Input: part model. Units: mm. Frame: model coordinates. A direction names the side the tool comes from. Give positions to 0.01 mm unless a question says otherwise; leave off trailing zeros. Loops run counter-clockwise (first coordinate to the right, second up) from the corner with the lowest first, then second, coordinate; pieces in that order, holes last. Notation, with made-up numbers: M 28,31 L 76,31 A12 ccw 76,53 Z; hole C -6,-24 d3. An arc over 180 degrees is marked long. Use CSV: the item, a comma, the result in double quotes. Start each with the question number.
Q1. Material intervals for line 1 along Z through (x, y) = (31, 13.5); line 2 along Y through (x, z) = (-48, 21.5); line 3 along Y through (x, z) = (-24, 26), sorted ascending.
Q2. Section B-B, the plane y = 25. Output: boundary loops of the cut face in (x, z).
Q3. Section A-A, the plane x = 0. Output: boundary loops of the cut face in (y, z), plus the area to 3 significant figures.
Q4. Section C-C, the plane x = 24. Output: boundary loops of the cut face in (y, z), plus the area to 3 significant figures.
Q5. Section D-D, the plane y = 3.5. Output: boundary loops of the cut face in (x, z) (3 decimals).
Q6. Pull-direction query (Z, two-part tool) for faces 1 (the flat face through (-1, 22, 16.95)), 2 (the cylindrical face through (-13.59, 1.01, 7.15)), 3 (the cylindrical face through (-46.06, 13.2, 20.52)), 4 (the flat face through (-2, 16, -24)); classes: released by +Z, released by -Z, zero draft, split by the parting line, or undercut.
Q7. Pin query (flat end, axial travel): pin 1 (3.5 mm diameter, centred on x = -14.94, z = -8.62, fed in from -Y); pin 2 (9 mm diameter, centred on x = -14.94, z = -8.62, fed in from +Y); pin 3 (6 mm diameter, centred on x = -24, y = 14, fed in from +Z). Return the tip coordinate at first contact, or that it passes through.
Q8. Reachability of faces 5 (the flat face through (-1, 36, 22)), 6 (the flat face through (-1, 7, -8)), 7 (the flat face through (27, 15.8, -25.5)), 8 (the cylindrical face through (-21.997, 14.631, 20.524)), 9 (the flat face through (-46, 12, 24)) from +Z, -Z, +X, -X, +Y, -Y: full face, straight path, thin tool, end or side. Return the list, or none.
from build123d import *

# Parameters (mm, degrees)
SKETCH1_W           = 108
SKETCH1_H           = 54
BOSS_EXTRUDE1_DEPTH = 6
SKETCH2_R           = 2
CUT_EXTRUDE1_DEPTH  = 12
SKETCH3_R           = 3.5
CUT_EXTRUDE3_DEPTH  = 4
SKETCH4_W           = 108
SKETCH4_H           = 54
BOSS_EXTRUDE2_DEPTH = 30
SKETCH5_W           = 108
SKETCH5_H           = 33.9
CUT_EXTRUDE4_DEPTH  = 29
SKETCH6_R           = 2.1
CUT_EXTRUDE5_DEPTH  = 67
SKETCH7_R           = 3.6
CUT_EXTRUDE6_DEPTH  = 3
CUT_EXTRUDE7_DEPTH  = 3
CUT_EXTRUDE8_START  = -3
SKETCH10_R          = 3.5
CUT_EXTRUDE8_DEPTH  = 3
SKETCH11_R          = 4
CUT_EXTRUDE9_DEPTH  = 10


with BuildPart() as part:
    # Sketch1 → Boss-Extrude1 (new body)
    with BuildSketch(Plane(origin=(0, 0, 0), x_dir=(1, 0, 0), z_dir=(0, 1, 0))):
        Rectangle(SKETCH1_W, SKETCH1_H)
    extrude(amount=BOSS_EXTRUDE1_DEPTH)

    # Sketch2 → Cut-Extrude1 (cut)
    with BuildSketch(Plane(origin=(0, 6, 0), x_dir=(1, 0, 0), z_dir=(0, 1, 0))):
        with Locations(Location((-14.938938215, 8.625, 0), (0, 0, 270))):
            Circle(SKETCH2_R)
        with Locations(Location((-14.938938215, -8.625, 0), (0, 0, 270))):
            Circle(SKETCH2_R)
        with Locations(Location((15.385610645, 7.800351601, 0), (0, 0, 270))):
            Circle(SKETCH2_R)
        with Locations(Location((15.385610645, -8.625, 0), (0, 0, 270))):
            Circle(SKETCH2_R)
    extrude(amount=-CUT_EXTRUDE1_DEPTH, mode=Mode.SUBTRACT)

    # Sketch3 → Cut-Extrude3 (cut)
    with BuildSketch(Plane(origin=(0, 6, 0), x_dir=(1, 0, 0), z_dir=(0, 1, 0))):
        with Locations(Location((-14.938938215, 8.625, 0), (0, 0, 270))):
            Circle(SKETCH3_R)
        with Locations(Location((-14.938938215, -8.625, 0), (0, 0, 270))):
            Circle(SKETCH3_R)
        with Locations(Location((15.385610645, 7.800351601, 0), (0, 0, 270))):
            Circle(SKETCH3_R)
        with Locations(Location((15.385610645, -8.625, 0), (0, 0, 270))):
            Circle(SKETCH3_R)
    extrude(amount=-CUT_EXTRUDE3_DEPTH, mode=Mode.SUBTRACT)

    # Sketch4 → Boss-Extrude2 (add)
    with BuildSketch(Plane(origin=(0, 6, 0), x_dir=(1, 0, 0), z_dir=(0, 1, 0))):
        Rectangle(SKETCH4_W, SKETCH4_H)
    extrude(amount=BOSS_EXTRUDE2_DEPTH)

    # Sketch5 → Cut-Extrude4 (cut)
    with BuildSketch(Plane(origin=(0, 36, 0), x_dir=(1, 0, 0), z_dir=(0, 1, 0))):
        Rectangle(SKETCH5_W, SKETCH5_H)
    extrude(amount=-CUT_EXTRUDE4_DEPTH, mode=Mode.SUBTRACT)

    # Sketch6 → Cut-Extrude5 (cut)
    with BuildSketch(Plane.XY.offset(27)):
        with Locations((0, 14)):
            Circle(SKETCH6_R)
        with Locations((-24, 14)):
            Circle(SKETCH6_R)
        with Locations((-48, 14)):
            Circle(SKETCH6_R)
        with Locations((24, 14)):
            Circle(SKETCH6_R)
        with Locations((48, 14)):
            Circle(SKETCH6_R)
        with Locations((48, 32)):
            Circle(SKETCH6_R)
        with Locations((-48, 32)):
            Circle(SKETCH6_R)
    extrude(amount=-CUT_EXTRUDE5_DEPTH, mode=Mode.SUBTRACT)

    # Sketch7 → Cut-Extrude6 (cut)
    with BuildSketch(Plane.XY.offset(27)):
        with Locations((-48, 32)):
            Circle(SKETCH7_R)
        with Locations((-48, 14)):
            Circle(SKETCH7_R)
        with Locations((-24, 14)):
            Circle(SKETCH7_R)
        with Locations((0, 14)):
            Circle(SKETCH7_R)
        with Locations((24, 14)):
            Circle(SKETCH7_R)
        with Locations((48, 14)):
            Circle(SKETCH7_R)
        with Locations((48, 32)):
            Circle(SKETCH7_R)
    extrude(amount=-CUT_EXTRUDE6_DEPTH, mode=Mode.SUBTRACT)

    # Sketch8 → Cut-Extrude7 (cut)
    with BuildSketch(Plane(origin=(0, 0, -27), x_dir=(-1, 0, 0), z_dir=(0, 0, -1))):
        Polygon((-50.020725942, 28.5), (-45.979274058, 28.5), (-43.958548116, 32), (-45.979274058, 35.5), (-50.020725942, 35.5), (-52.041451884, 32), align=None)
        Polygon((-50.020725942, 10.5), (-45.979274058, 10.5), (-43.958548116, 14), (-45.979274058, 17.5), (-50.020725942, 17.5), (-52.041451884, 14), align=None)
        Polygon((-26.020725942, 10.5), (-21.979274058, 10.5), (-19.958548116, 14), (-21.979274058, 17.5), (-26.020725942, 17.5), (-28.041451884, 14), align=None)
        Polygon((-2.020725942, 10.5), (2.020725942, 10.5), (4.041451884, 14), (2.020725942, 17.5), (-2.020725942, 17.5), (-4.041451884, 14), align=None)
        Polygon((21.979274058, 10.5), (26.020725942, 10.5), (28.041451884, 14), (26.020725942, 17.5), (21.979274058, 17.5), (19.958548116, 14), align=None)
        Polygon((45.979274058, 10.5), (50.020725942, 10.5), (52.041451884, 14), (50.020725942, 17.5), (45.979274058, 17.5), (43.958548116, 14), align=None)
        Polygon((45.979274058, 28.5), (50.020725942, 28.5), (52.041451884, 32), (50.020725942, 35.5), (45.979274058, 35.5), (43.958548116, 32), align=None)
    extrude(amount=-CUT_EXTRUDE7_DEPTH, mode=Mode.SUBTRACT)

    # Sketch10 → Cut-Extrude8 (cut)
    with BuildSketch(Plane.XZ.offset(-6).offset(CUT_EXTRUDE8_START)):
        with Locations(Location((-14.938938215, -8.625, 0), (0, 0, 90))):
            Circle(SKETCH10_R)
        with Locations(Location((-14.938938215, 8.625, 0), (0, 0, 90))):
            Circle(SKETCH10_R)
        with Locations(Location((15.385610645, 8.625, 0), (0, 0, 90))):
            Circle(SKETCH10_R)
        with Locations(Location((15.385610645, -7.800351601, 0), (0, 0, 90))):
            Circle(SKETCH10_R)
    extrude(amount=CUT_EXTRUDE8_DEPTH, mode=Mode.SUBTRACT)

    # Sketch11 → Cut-Extrude9 (cut)
    with BuildSketch(Plane(origin=(0, 7, 0), x_dir=(1, 0, 0), z_dir=(0, 1, 0))):
        with Locations(Location((0, 0, 0), (0, 0, 270))):
            Circle(SKETCH11_R)
    extrude(amount=-CUT_EXTRUDE9_DEPTH, mode=Mode.SUBTRACT)


solid = part.part
A:
1,line 1,"-27 to -16.95, 16.95 to 27"
1,line 2,"0 to 11.9, 16.1 to 29.9, 34.1 to 36"
1,line 3,"0 to 10.4, 17.6 to 36"
2,outline,"M -54,-27 L 54,-27 L 54,-16.95 L -54,-16.95 Z; M -54,16.95 L 54,16.95 L 54,27 L -54,27 Z"
3,outline,"M 0,-27 L 10.5,-27 L 10.5,-24 L 11.9,-24 L 11.9,-16.95 L 7,-16.95 L 7,-4 L 0,-4 Z; M 0,4 L 7,4 L 7,16.95 L 11.9,16.95 L 11.9,24 L 10.4,24 L 10.4,27 L 0,27 Z; M 16.1,-24 L 17.5,-24 L 17.5,-27 L 36,-27 L 36,-16.95 L 16.1,-16.95 Z; M 16.1,16.95 L 36,16.95 L 36,27 L 17.6,27 L 17.6,24 L 16.1,24 Z"
3,area,"803 mm^2"
4,outline,"M 0,-27 L 10.5,-27 L 10.5,-24 L 11.9,-24 L 11.9,-16.95 L 7,-16.95 L 7,16.95 L 11.9,16.95 L 11.9,24 L 10.4,24 L 10.4,27 L 0,27 Z; M 16.1,-24 L 17.5,-24 L 17.5,-27 L 36,-27 L 36,-16.95 L 16.1,-16.95 Z; M 16.1,16.95 L 36,16.95 L 36,27 L 17.6,27 L 17.6,24 L 16.1,24 Z"
4,area,"859 mm^2"
5,outline,"M -54,-27 L 54,-27 L 54,27 L -54,27 Z; hole C -14.939,-8.625 d7; hole C -14.939,8.625 d7; hole C 0,0 d8; hole C 15.386,-7.8 d7; hole C 15.386,8.625 d7"
6,face 1,"undercut"
6,face 2,"undercut"
6,face 3,"zero draft"
6,face 4,"released by -Z"
7,pin 1,"through"
7,pin 2,"y = 7"
7,pin 3,"z = 24"
8,face 5,"+Z, -Z, +X, -X, +Y"
8,face 6,"+X, -X, +Y"
8,face 7,"-Z"
8,face 8,"+Z, -Z"
8,face 9,"+Z"
